For this review, take the finished solid that the model builds, in its own axes (mm). A direction names the side the tool comes from. Give positions to 0.01 mm unless a question says otherwise; leave off trailing zeros. Loops run counter-clockwise (first coordinate to the right, second up) from the corner with the lowest first, then second, coordinate; pieces in that order, holes last.
```python
from build123d import *

# Parameters (mm, degrees)
SKETCH_W     = 90
SKETCH_H     = 10
SKETCH_R     = 2
PAD_DEPTH    = 2.5
PAD001_DEPTH = 26
PAD002_DEPTH = 2


with BuildPart() as part:
    # Sketch → Pad (new body)
    with BuildSketch(Plane.XY):
        Rectangle(SKETCH_W, SKETCH_H)
        with Locations((-40, 0)):
            Circle(SKETCH_R, mode=Mode.SUBTRACT)
        with Locations((40, 0)):
            Circle(SKETCH_R, mode=Mode.SUBTRACT)
    extrude(amount=PAD_DEPTH)

    # Sketch001 → Pad001 (new body)
    with BuildSketch(Plane.XY.offset(2.5)):
        with BuildLine():
            ThreePointArc((35, -5.068991), (0, 4.896818), (-35, -5.068991))
            Line((-35, -5.068991), (35, -5.068991))
        make_face()
    extrude(amount=PAD001_DEPTH)

    # Sketch002 → Pad002 (new body)
    with BuildSketch(Plane.XY.offset(28.5)):
        with BuildLine():
            ThreePointArc((35, 10), (0, 23.686319), (-35, 10))
            Line((-35, -5), (-35, 10))
            Line((-35, -5), (35, -5))
            Line((35, 10), (35, -5))
        make_face()
    extrude(amount=PAD002_DEPTH)


solid = part.part
```
Q1. Consider section D-D on x = -18. Give the boundary of the cut face in (y, z).
Answers:
outline: (-5.07, 2.5) - (-5, 2.5) - (-5, 0) - (5, 0) - (5, 2.5) - (2.41, 2.5) - (2.41, 28.5) - (20.44, 28.5) - (20.44, 30.5) - (-5, 30.5) - (-5, 28.5) - (-5.07, 28.5) - close
Q2. Consider section B-B on y = 0. Give the boundary of the cut face in (x, z).
Answers:
outline: (-45, 0) - (-42, 0) - (-42, 2.5) - (-45, 2.5) - close; (-38, 0) - (38, 0) - (38, 2.5) - (25.03, 2.5) - (25.03, 28.5) - (35, 28.5) - (35, 30.5) - (-35, 30.5) - (-35, 28.5) - (-25.03, 28.5) - (-25.03, 2.5) - (-38, 2.5) - close; (42, 0) - (45, 0) - (45, 2.5) - (42, 2.5) - close
Q3. Consider section C-C on z = 29.5. Give the boundary of the cut face in (x, y), plus the area to 3 significant figures.
Answers:
outline: (-35, -5) - (35, -5) - (35, 10) arc R51.6 ccw to (-35, 10) - close
area: 1,710 mm2
Q4. For pin 1 Ø6 at (x, z) = (-31, 17.5) entering from +Y; pin 2 Ø2 at (y, z) = (0.5, 29.5) entering from -X; pin 3 Ø1.2 at (x, z) = (-5, 1) entering from -Y, all flat-tipped, find the tip position at first contact; note any pin that passes through.
Answers:
pin 1: stops at y = -1.29
pin 2: stops at x = -35
pin 3: stops at y = -5
Q5. For probe 1 along Z at (x, y) = (-20, 3); probe 2 along Y at (x, z) = (40, 1.3); probe 3 along Z at (x, y) = (-21.5, 9.75), list the stretches that pass through material, from the lowest coordinate up.
Answers:
probe 1: z = 0 to 2.5, 28.5 to 30.5
probe 2: y = -5 to -2, 2 to 5
probe 3: z = 28.5 to 30.5
Q6. Consider section A-A on x = -40. Give the boundary of the cut face in (y, z), plus the area to 3 significant figures.
Answers:
outline: (-5, 0) - (-2, 0) - (-2, 2.5) - (-5, 2.5) - close; (2, 0) - (5, 0) - (5, 2.5) - (2, 2.5) - close
area: 15.0 mm2
Q7. Mouldability with a two-part tool opening along X and no side actions: class faces 4 (the cylindrical face through (-42, 0, 1)), 5 (the cylindrical face through (38, 0, 1)), 6 (the flat face through (-45, 0, 1)), 7 (the flat face through (-1, 5, 1)) as +X half, -X half, draft (parallel to the pull), parting line (faces both ways), or undercut.
Answers:
face 4: undercut
face 5: undercut
face 6: -X half
face 7: draft
Q8. Machinability: for faces 1 (the flat face through (-1, -5, 1)), 2 (the flat face through (35, 3, 29)), 3 (the cylindrical face through (0.516, 4.895, 15.318)), which of the approach directions +Z, -Z, +X, -X, +Y, -Y give a long, thin tool a straight path to every point of the face, cutting with its end or side? Answer none if there is none.
Answers:
face 1: -Z, +X, -X, -Y
face 2: +Z, +X, +Y, -Y
face 3: +Y
